Job drawing, mm, ordinate dimensions from the low corner. One solid piece. Round coordinates to 2 decimals unless told otherwise and drop trailing zeros. Write each loop counter-clockwise with the first axis right and the second up, starting at its lowest first coordinate (ties: lowest second). Pieces come first, ordered by that corner, then holes.
1) Pull direction Y, two halves, no side cores. Call the marked faces 1, 2 and 3: +Y half, -Y half, draft (parallel to the pull), parting line (faces both ways), or undercut.
2) Drill centre lines: L1, parallel to X at y = 3.25, z = 0.6; L2, parallel to X at y = 3.25, z = 1.6 (1 decimal); L3, parallel to Y at x = 2.8, z = 0.1 (1 decimal). Where is each one in solid material? Low to high.
3) Flat gauge pin, fed straight in: pin 1 (2 mm diameter, centred on x = 2.75, y = 3.18, fed in from -Z) (3 decimals). Where does the tip first touch, or does it go through?
4) Saw through at D-D on x = 4.55. Write the cut outline in (y, z).
5) Saw through at B-B on y = 1. Write the cut outline in (x, z).
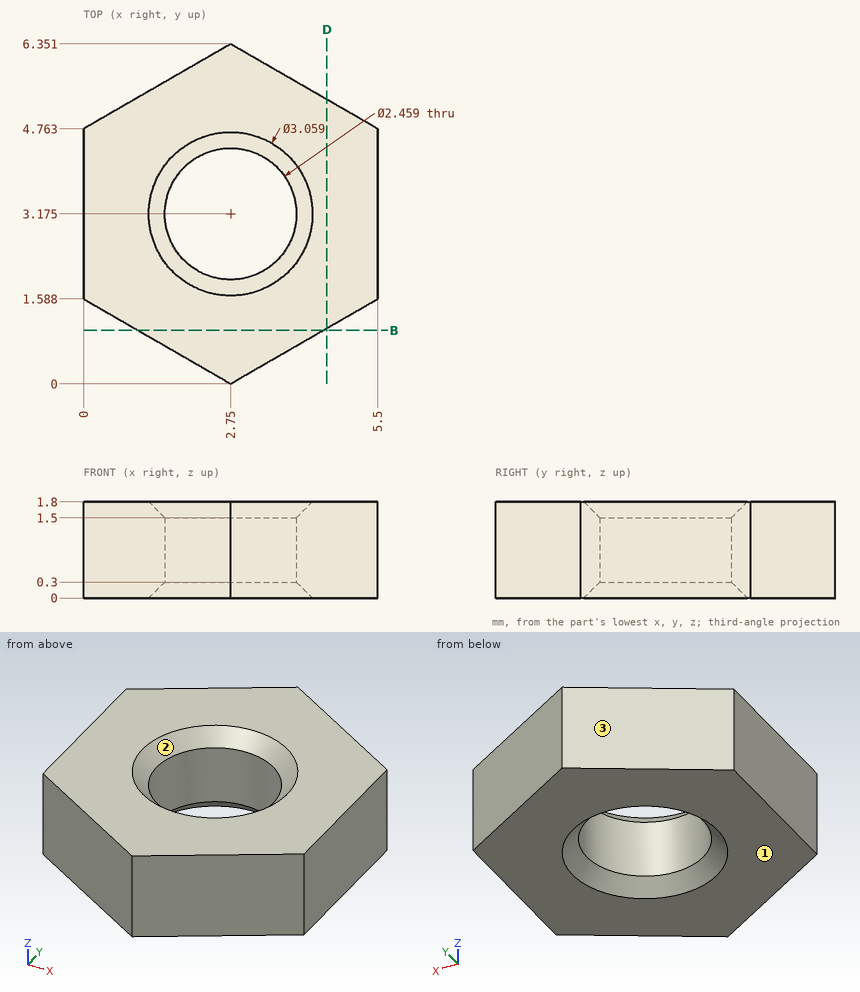
Completed:
1. face 1: draft
1. face 2: undercut
1. face 3: +Y half
2. L1: x = 0 to 1.52, 3.98 to 5.5
2. L2: x = 0 to 1.4, 4.1 to 5.5
2. L3: y = 0 to 1.7, 4.6 to 6.3
3. pin 1: passes through
4. outline: (1.04, 0) - (5.31, 0) - (5.31, 1.8) - (1.04, 1.8) - close
5. outline: (1.02, 0) - (4.48, 0) - (4.48, 1.8) - (1.02, 1.8) - close
